Build history of the part. All positions in model axes, mm. A direction names the side the tool comes from. Round coordinates to 2 decimals unless told otherwise and drop trailing zeros. Order: outer loops, then holes, each group sorted by start corner. A loop starts at its lowest first (then second) coordinate and runs counter-clockwise, first axis right, second up. Notation, with made-up numbers: M 65,69 L 74,69 A19 ccw 74,88 Z; hole C 8,-23.75 d1. An arc over 180 degrees is marked long. One line per item, written item: value. Start each with the question number.
Item 1: Tool access for faces 1 (the cylindrical face through (-12.932, 15.48, 5.362)), 2 (the flat face through (-2, 42.4, -2)): list every direction of +Z, -Z, +X, -X, +Y, -Y with a clear straight run to the whole face (end or side of a thin tool).
Item 2: Band-saw the part on D-D, the plane z = 72.5. Write the cut outline in (x, y).
Item 3: Band-saw the part on C-C, the plane y = 10. Write the cut outline in (x, z).
Item 4: Two-plate mould, pull along Y, no slides. Class faces 3 (the cylindrical face through (73.113, 37.963, -114.676)), 4 (the flat face through (0, 31.4, -6)), 5 (the flat face through (0, 0, 0)), 6 (the cylindrical face through (-1.19, 32.39, -5.37)): +Y half, -Y half, draft (parallel to the pull), parting line (faces both ways), or undercut.
Item 5: Probe L1, parallel to Y at x = 111, z = 53; L2, parallel to X at y = 11, z = -3; L3, parallel to X at y = 37.5, z = -41.5. List the from-to ranges inside material, lowest first.
Item 6: Pin check, flat tips, straight feed: pin 1 (12 mm diameter, centred on x = 25.5, y = 24.5, fed in from -Z); pin 2 (4 mm diameter, centred on y = 34.5, z = -59.5, fed in from -X); pin 3 (2 mm diameter, centred on x = -92, z = 11, fed in from -Y); pin 4 (8 mm diameter, centred on y = 23, z = -4, fed in from +X). Stop position of each tip, or through.
Item 7: Band-saw the part on A-A, the plane z = 0. Write the cut outline in (x, y).
Item 8: Band-saw the part on B-B, the plane x = 0. Write the cut outline in (y, z).
Autodesk Inventor part; units mm, degrees
ref_plane "YZ Plane" through (0, 0, 0) normal (1, 0, 0) x (0, 1, 0)
ref_plane "XZ Plane" through (0, 0, 0) normal (0, 1, 0) x (-1, 0, 0)
ref_plane "XY Plane" through (0, 0, 0) normal (0, 0, 1) x (1, 0, 0)
sketch "Sketch1" plane through (0, 0, 0) normal (0, 1, 0) x (-1, 0, 0)
  circle A0 centre (0, 0) radius 14
  dimension "d0" = 28
extrude "Extrusion1" add sketch "Sketch1" along normal blind 31.4
sketch "Sketch2" plane through (0, 31.4, 0) normal (0, 1, 0) x (1, 0, 0)
  circle A0 centre (0, 0) radius 5.5
  dimension "d3" = 11
extrude "Extrusion2" add sketch "Sketch2" along normal blind 11
sketch "Sketch3" plane through (0, 42.4, 0) normal (0, 1, 0) x (1, 0, 0)
  circle A0 centre (0, 0) radius 14
  circle A1 centre (0, 0) radius 136
  dimension "d6" = 272
extrude "Extrusion3" add sketch "Sketch3" against normal blind 9 contours A0 | A1
properties part number "motor_with_prop"
Output:
1. face 1: -Y
1. face 2: +Z, -Z, +X, -X, +Y
2. outline: M -115.06,33.4 L 115.06,33.4 L 115.06,42.4 L -115.06,42.4 Z
3. outline: C 0,0 d28
4. face 3: draft
4. face 4: undercut
4. face 5: -Y half
4. face 6: undercut
5. L1: y = 33.4 to 42.4
5. L2: x = -13.67 to 13.67
5. L3: x = -129.51 to 129.51
6. pin 1: passes through
6. pin 2: stops at x = -123.25
6. pin 3: stops at y = 33.4
6. pin 4: stops at x = 14
7. outline: M -136,33.4 L -5.5,33.4 L -5.5,31.4 L -14,31.4 L -14,0 L 14,0 L 14,31.4 L 5.5,31.4 L 5.5,33.4 L 136,33.4 L 136,42.4 L -136,42.4 Z
8. outline: M 0,-14 L 31.4,-14 L 31.4,-5.5 L 33.4,-5.5 L 33.4,-136 L 42.4,-136 L 42.4,136 L 33.4,136 L 33.4,5.5 L 31.4,5.5 L 31.4,14 L 0,14 Z
